from build123d import *

# Parameters (mm, degrees)
SKETCH2_R               = 50.875
SKETCH2_R_2             = 47.875
BOSS_EXTRUDE1_DEPTH     = 60
CUT_EXTRUDE2_DEPTH      = 60
CUT_EXTRUDE2_DEPTH_BACK = 60
SKETCH3_OUTSIDE_W       = 93.18
SKETCH3_OUTSIDE_H       = 134.93
CUT_EXTRUDE3_DEPTH      = 94.683142827
CUT_EXTRUDE3_DEPTH_BACK = 94.683142827
SKETCH4_R               = 4.765
FILLET1_R               = 20
SKETCH5_W               = 5
SKETCH5_H               = 5
CUT_EXTRUDE4_DEPTH      = 60


with BuildPart() as part:
    # Sketch2 → Boss-Extrude1 (new body)
    with BuildSketch(Plane.XY):
        with Locations(Location((0, 0, 0), (0, 0, 180))):
            Circle(SKETCH2_R)
        with Locations(Location((0, 0, 0), (0, 0, 180))):
            Circle(SKETCH2_R_2, mode=Mode.SUBTRACT)
    extrude(amount=BOSS_EXTRUDE1_DEPTH)

    # Sketch3 outside → Cut-Extrude2 (cut, two sides: drawn at the far end of the back side and taken through both)
    with BuildSketch(Plane(origin=(0, 0, 0), x_dir=(0, 0, -1), z_dir=(1, 0, 0)).offset(-CUT_EXTRUDE2_DEPTH_BACK)):
        with Locations((-30, 0)):
            Rectangle(SKETCH3_OUTSIDE_W, SKETCH3_OUTSIDE_H)
        Polygon((-60, 50.875), (-60, -50.875), (0, -50.875), (0, 15.646937383), (-30, 15.646937383), (-30, 50.875), align=None, mode=Mode.SUBTRACT)
    extrude(amount=CUT_EXTRUDE2_DEPTH + CUT_EXTRUDE2_DEPTH_BACK, mode=Mode.SUBTRACT)

    # Sketch4 → Cut-Extrude3 (cut, two sides: drawn at the far end of the back side and taken through both)
    with BuildSketch(Plane(origin=(0, 0, 0), x_dir=(0, 0, -1), z_dir=(1, 0, 0)).offset(-CUT_EXTRUDE3_DEPTH_BACK)):
        with Locations((-17, 0)):
            Circle(SKETCH4_R)
    extrude(amount=CUT_EXTRUDE3_DEPTH + CUT_EXTRUDE3_DEPTH_BACK, mode=Mode.SUBTRACT)

    # Fillet1
    # the kernel refuses this fillet: 20 mm, written as the material it takes off along each edge
    with BuildSketch(Plane(origin=(-4.75412753, 15.646937383, 0), x_dir=(0, -1, 0), z_dir=(1, 0, 0)), Plane(origin=(-98.409079474, 15.646937383, 0), x_dir=(0, -1, 0), z_dir=(1, 0, 0))) as fillet1_piece_1:
        with BuildLine():
            CenterArc((FILLET1_R, -FILLET1_R), FILLET1_R, 90, 90)
            Line((0, -FILLET1_R), (0, 0))
            Line((0, 0), (FILLET1_R, 0))
        make_face()
    extrude(amount=103.163207005, mode=Mode.SUBTRACT)

    # Sketch5 → Cut-Extrude4 (cut)
    with BuildSketch(Plane(origin=(0, 0, 0), x_dir=(1, 0, 0), z_dir=(0, 1, 0))):
        with Locations((0, -60)):
            Rectangle(SKETCH5_W, SKETCH5_H)
    extrude(amount=CUT_EXTRUDE4_DEPTH, mode=Mode.SUBTRACT)


solid = part.part
The model under review builds one solid part; all positions refer to its coordinate system, in mm. A direction names the side the tool comes from. Round coordinates to 2 decimals unless told otherwise and drop trailing zeros. Loops run counter-clockwise (first coordinate to the right, second up) from the corner with the lowest first, then second, coordinate; pieces in that order, holes last. Notation, with made-up numbers: M 24.25,-28.5 L 43.25,-28.5 A15 ccw 43.25,-0.5 Z; hole C 87.25,-33.5 d7. An arc over 180 degrees is marked long. Answer as CSV lines item,"result". Start each with the question number.
Item 1: Consider section A-A (x = 0). Write out the cut boundary in (y, z) (3 decimals).
Item 2: Consider section C-C (y = 0). Write out the cut boundary in (x, z) (3 decimals).
Item 3: For faces 5 (the face through (-2.5, 49, 59)), 6 (the face through (0, 49, 30)), 7 (the face through (0.2, -48.4, 0)), list the 3-axis set-ups (+Z, -Z, +X, -X, +Y, -Y) from which the entire face can be reached by the end or side of a thin tool; tool diameter is ignored.
Item 4: Consider section D-D (y = -34.5). Write out the cut boundary in (x, z).
Item 5: Mouldability with a two-part tool opening along X and no side actions: class faces 1 (the face through (2.5, 49, 59)), 2 (the face through (47, 15.647, 25)), 3 (the face through (0, 49, 57.5)), 4 (the face through (6.623, -50.442, 36.247)) as released by +X, released by -X, zero draft, split by the parting line, or undercut.
Item 6: Consider section B-B (z = 17). State how many separate pieces and enclosed holes the cut face has, then the cut area to 3 significant figures.
Item 7: Wall thickness on line 1 (Y direction, x = -6, z = 49); line 2 (X direction, y = -8, z = 35); line 3 (Y direction, x = 0, z = 37) (3 decimals): over which ranges is each line inside the solid? List them lowest first. Write a range as [from, to].
Item 8: Insertion check: P1, Ø1.6, axis at x = 46.5, z = 26.5, coming from the +Y side; P2, Ø1, axis at x = -24.5, z = 20.5, coming from the -Y side; P3, Ø12, axis at x = 12.5, z = 50.5, coming from the +Y side. Each pin has a flat end and moves straight along its axis. Give the tip position at first contact, or say it passes through.
Answer:
1,outline,"M -50.875,0 L -47.875,0 L -47.875,60 L -50.875,60 Z; M 47.875,30 L 50.875,30 L 50.875,57.5 L 47.875,57.5 Z"
2,outline,"M -50.875,0.479 L -47.875,0.479 L -47.875,12.235 L -50.875,12.235 Z; M -50.875,21.765 L -47.875,21.765 L -47.875,60 L -50.875,60 Z; M 47.875,0.479 L 50.875,0.479 L 50.875,12.235 L 47.875,12.235 Z; M 47.875,21.765 L 50.875,21.765 L 50.875,60 L 47.875,60 Z"
3,face 5,"+Z, +Y"
3,face 6,"-Z, +X, -X, +Y"
3,face 7,"-Z, +X, -X, +Y, -Y"
4,outline,"M -37.39,0 L -33.19,0 L -33.19,60 L -37.39,60 Z; M 33.19,0 L 37.39,0 L 37.39,60 L 33.19,60 Z"
5,face 1,"undercut"
5,face 2,"zero draft"
5,face 3,"undercut"
5,face 4,"split by the parting line"
6,separate pieces,"3"
6,enclosed holes,"0"
6,area,"502 mm^2"
7,line 1,"y = [-50.52, -47.5], [47.5, 50.52]"
7,line 2,"x = [-50.24, -47.2], [47.2, 50.24]"
7,line 3,"y = [-50.875, -47.875], [47.875, 50.875]"
8,P1,"stops at y = 15.65"
8,P2,"stops at y = -44.86"
8,P3,"stops at y = 50.46"
